Work out the finished part from the listing and answer in its coordinate system (mm). A direction names the side the tool comes from. Coordinates: 2 decimals unless noted, no trailing zeros. Write each loop counter-clockwise with the first axis right and the second up, starting at its lowest first coordinate (ties: lowest second). Pieces come first, ordered by that corner, then holes. Notation, with made-up numbers: M -2,26.5 L 19,26.5 A24 ccw 19,45.5 Z; hole C 34.5,83.25 d9. An arc over 180 degrees is marked long. Answer as CSV lines item,"result". Start each with the question number.
(1) A cutting plane is placed at B-B on y = -25. Give the vertices of the cut face in (x, z), then the cut area to 3 significant figures.
(2) A cutting plane is placed at D-D on y = 79.5. Give the vertices of the cut face in (x, z), then the cut area to 3 significant figures.
(3) The mould has two halves that part along Y. Classify faces 4 (the flat face through (90, 58.881, 40)), 5 (the flat face through (88, 96.141, 18)), 6 (the flat face through (90, 78, 53.086)): released by +Y, released by -Y, zero draft, split by the parting line, or undercut.
(4) For faces 1 (the flat face through (90, -49.571, 40)), 2 (the flat face through (27.452, -69, 40)), 3 (the flat face through (88, -88.466, 31)), determine the directions among +Z, -Z, +X, -X, +Y, -Y from which every point of the face is accessible in a straight line to the end or side of a thin tool.
(5) A cutting plane is placed at A-A on z = 40.5. Give the vertices of the cut face in (x, y), then the cut area to 3 significant figures.
(6) Find the intervals of material crossed by L1, parallel to Z at x = -149.5, y = -21.5; L2, parallel to Y at x = 156.5, z = 20.5; L3, parallel to X at y = -32, z = 27.5, in increasing order. Write a range as [from, to].
(7) A cutting plane is placed at C-C on x = 53.5. Give the vertices of the cut face in (y, z), then the cut area to 3 significant figures.
(8) Flat-ended cylindrical pins translate along their axes: P1, Ø12, axis at x = 17, y = -15, coming from the -Z side; P2, Ø6, axis at y = 79, z = 18, coming from the +X side; P3, Ø14, axis at y = -37.5, z = 20.5, coming from the -X side; P4, Ø7.5, axis at y = -69, z = 36, coming from the -X side. Find the tip coordinate at first contact, or state that the pin passes through.
from build123d import *

# Parameters (mm, degrees)
F1_W      = 179.506913
F1_H      = 184.607744
F2_DEPTH  = 14.986
F2_FACE_W = 179.506912
F2_FACE_H = 184.607744
F3_DEPTH  = 12.7
F4_W      = 126.293604
F4_H      = 37.260275
F4_H_2    = 38.89557
F5_DEPTH  = 25.4
F0_W      = 363.899439
F0_H      = 194.727853
F6_DEPTH  = 9.398


with BuildPart() as f2:
    # F1 (on face) → F2 (new body)
    with BuildSketch(Plane.XY):
        with Locations((89.753456, 3.837615)):
            Rectangle(F1_W, F1_H)
    extrude(amount=F2_DEPTH)

    # F2_face (on face) → F3 (join, symmetric)
    with BuildSketch(Plane(origin=(89.753456, 3.837615, 14.986), x_dir=(1, 0, 0), z_dir=(0, 0, 1))):
        Rectangle(F2_FACE_W, F2_FACE_H)
    extrude(amount=F3_DEPTH, both=True)

    # F4 (on face) → F5 (join)
    with BuildSketch(Plane.XY.offset(27.686)):
        with Locations((90.598954, 77.511349)):
            Rectangle(F4_W, F4_H)
        with Locations((90.598954, -69.018472)):
            Rectangle(F4_W, F4_H_2)
    extrude(amount=F5_DEPTH)

    # F0 (on Top) → F6 (join)
    with BuildSketch(Plane.XY):
        with Locations((1.610697, 3.912329)):
            Rectangle(F0_W, F0_H)
    extrude(amount=F6_DEPTH)


solid = f2.part
Here are the results:
1,outline,"M -180.34,0 L 183.56,0 L 183.56,9.4 L 179.51,9.4 L 179.51,27.69 L 0,27.69 L 0,9.4 L -180.34,9.4 Z"
1,area,"6,700 mm^2"
2,outline,"M -180.34,0 L 183.56,0 L 183.56,9.4 L 179.51,9.4 L 179.51,27.69 L 153.75,27.69 L 153.75,53.09 L 27.45,53.09 L 27.45,27.69 L 0,27.69 L 0,9.4 L -180.34,9.4 Z"
2,area,"9,910 mm^2"
3,face 4,"undercut"
3,face 5,"released by +Y"
3,face 6,"zero draft"
4,face 1,"+Z, +X, -X"
4,face 2,"+Z, -X, +Y, -Y"
4,face 3,"+Z, +X, -X, -Y"
5,outline,"M 27.45,-88.47 L 153.75,-88.47 L 153.75,-49.57 L 27.45,-49.57 Z; M 27.45,58.88 L 153.75,58.88 L 153.75,96.14 L 27.45,96.14 Z"
5,area,"9,620 mm^2"
6,L1,"z = [0, 9.4]"
6,L2,"y = [-88.47, 96.14]"
6,L3,"x = [0, 179.51]"
7,outline,"M -93.45,0 L 101.28,0 L 101.28,9.4 L 96.14,9.4 L 96.14,53.09 L 58.88,53.09 L 58.88,27.69 L -49.57,27.69 L -49.57,53.09 L -88.47,53.09 L -88.47,9.4 L -93.45,9.4 Z"
7,area,"7,140 mm^2"
8,P1,"stops at z = 0"
8,P2,"stops at x = 179.51"
8,P3,"stops at x = 0"
8,P4,"stops at x = 27.45"
